The model under review builds one solid part; all positions refer to its coordinate system, in mm. A direction names the side the tool comes from. Coordinates: 2 decimals unless noted, no trailing zeros. Write each loop counter-clockwise with the first axis right and the second up, starting at its lowest first coordinate (ties: lowest second). Pieces come first, ordered by that corner, then holes. Notation, with made-up numbers: M 8,-36.5 L 46,-36.5 A12 ccw 46,-32.5 Z; hole C 64,-7.75 d9. An arc over 180 degrees is marked long. Answer as a JSON object with one key per item and string values.
```python
from build123d import *

# Parameters (mm, degrees)
SKETCH1_W           = 177.8
SKETCH1_H           = 177.8
BOSS_EXTRUDE1_DEPTH = 12.7
BOSS_EXTRUDE2_DEPTH = 76.2


with BuildPart() as part:
    # Sketch1 → Boss-Extrude1 (new, symmetric)
    with BuildSketch(Plane(origin=(0, 0, 0), x_dir=(1, 0, 0), z_dir=(0, 1, 0))):
        Rectangle(SKETCH1_W, SKETCH1_H)
    extrude(amount=BOSS_EXTRUDE1_DEPTH, both=True)

    # Sketch2 → Boss-Extrude2 (add, symmetric)
    with BuildSketch(Plane(origin=(0, 0, 0), x_dir=(0, 0, -1), z_dir=(1, 0, 0))):
        with BuildLine():
            Line((-38.1, -25.4), (-38.1, 50.8))
            ThreePointArc((-38.1, 50.8), (0, 88.9), (38.1, 50.8))
            Line((38.1, 50.8), (38.1, -25.4))
            ThreePointArc((38.1, -25.4), (0, -63.5), (-38.1, -25.4))
        make_face()
    extrude(amount=BOSS_EXTRUDE2_DEPTH, both=True)


solid = part.part
```
(1) For pin 1 Ø6 at (y, z) = (44, 5) entering from +X; pin 2 Ø8 at (x, y) = (45.5, -24) entering from -Z; pin 3 Ø10 at (x, z) = (-41.5, 29.5) entering from -Y, all flat-tipped, find the tip position at first contact; note any pin that passes through.
Results list:
{"pin 1": "x = 76.2", "pin 2": "z = -38.1", "pin 3": "y = -54.58"}
(2) Add section B-B on x = 31. Give the boundary of the cut face in (y, z).
Results list:
{"outline": "M -25.4,-38.1 L -12.7,-38.1 L -12.7,-88.9 L 12.7,-88.9 L 12.7,-38.1 L 50.8,-38.1 A38.1 ccw 50.8,38.1 L 12.7,38.1 L 12.7,88.9 L -12.7,88.9 L -12.7,38.1 L -25.4,38.1 A38.1 ccw Z"}
(3) Add section C-C on y = 33. Give the boundary of the cut face in (x, z), and give its area (3 significant figures).
Results list:
{"outline": "M -76.2,-38.1 L 76.2,-38.1 L 76.2,38.1 L -76.2,38.1 Z", "area": "11,600 mm²"}
(4) Wall thickness on line 1 along Y through (x, z) = (-34, 40.5); line 2 along X through (y, z) = (56.5, -16); line 3 along Z through (x, y) = (-18, -25): over which ranges is each line inside the solid? List them lowest first. Write a range as from..to.
Results list:
{"line 1": "-12.7..12.7", "line 2": "-76.2..76.2", "line 3": "-38.1..38.1"}
(5) For faces 1 (the face through (-76.2, -32, -1)), 2 (the face through (1, -19, 38.1)), 3 (the face through (1, -19, -38.1)), 4 (the face through (1, 31, 38.1)), list the 3-axis set-ups (+Z, -Z, +X, -X, +Y, -Y) from which the entire face can be reached by the end or side of a thin tool; tool diameter is ignored.
Results list:
{"face 1": "+Z, -Z, -X, -Y", "face 2": "+Z, +X, -X, -Y", "face 3": "-Z, +X, -X, -Y", "face 4": "+Z, +X, -X, +Y"}
(6) Add section A-A on z = 0. Give the boundary of the cut face in (x, y), and give its area (3 significant figures).
Results list:
{"outline": "M -88.9,-12.7 L -76.2,-12.7 L -76.2,-63.5 L 76.2,-63.5 L 76.2,-12.7 L 88.9,-12.7 L 88.9,12.7 L 76.2,12.7 L 76.2,88.9 L -76.2,88.9 L -76.2,12.7 L -88.9,12.7 Z", "area": "23,900 mm²"}
(7) Add section D-D on z = -72. Give the boundary of the cut face in (x, y).
Results list:
{"outline": "M -88.9,-12.7 L 88.9,-12.7 L 88.9,12.7 L -88.9,12.7 Z"}
